```python
from build123d import *

# Parameters (mm, degrees)
SKETCH_1_W          = 20
SKETCH_1_H          = 20
EXTRUDE_1_DEPTH     = 50
SKETCH_2_R          = 1.5
CUT_EXTRUDE_1_DEPTH = 20
SKETCH_4_R          = 1.5
CUT_EXTRUDE_3_DEPTH = 20


with BuildPart() as part:
    # 草图1 → 凸台-拉伸1 (new body)
    with BuildSketch(Plane.XY):
        Rectangle(SKETCH_1_W, SKETCH_1_H)
    extrude(amount=EXTRUDE_1_DEPTH)

    # 草图2 → 切除-拉伸1 (cut)
    with BuildSketch(Plane(origin=(10, 0, 0), x_dir=(0, 0, -1), z_dir=(1, 0, 0))):
        with Locations((-32.5, 5.05)):
            Circle(SKETCH_2_R)
        with Locations((-17.5, 5.05)):
            Circle(SKETCH_2_R)
        with Locations((-32.5, -4.95)):
            Circle(SKETCH_2_R)
        with Locations((-17.5, -4.95)):
            Circle(SKETCH_2_R)
    extrude(amount=-CUT_EXTRUDE_1_DEPTH, mode=Mode.SUBTRACT)

    # 草图4 → 切除-拉伸3 (cut)
    with BuildSketch(Plane.XZ.offset(10)):
        with Locations(Location((-4.85, 40.893026958, 0), (0, 0, 270))):
            Circle(SKETCH_4_R)
        with Locations(Location((-4.85, 24.893026958, 0), (0, 0, 270))):
            Circle(SKETCH_4_R)
        with Locations(Location((-4.85, 8.893026958, 0), (0, 0, 270))):
            Circle(SKETCH_4_R)
        with Locations(Location((4.85, 8.893026958, 0), (0, 0, 270))):
            Circle(SKETCH_4_R)
        with Locations(Location((4.85, 24.893026958, 0), (0, 0, 270))):
            Circle(SKETCH_4_R)
        with Locations(Location((4.85, 40.893026958, 0), (0, 0, 270))):
            Circle(SKETCH_4_R)
    extrude(amount=-CUT_EXTRUDE_3_DEPTH, mode=Mode.SUBTRACT)


solid = part.part
```
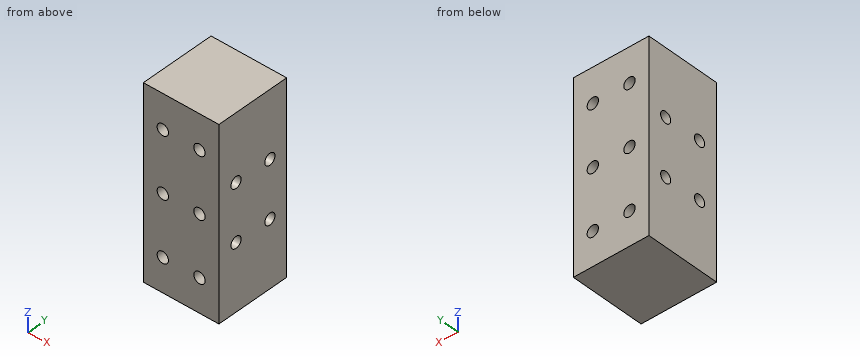
The listing builds one solid part. Answer for the finished solid, in the listing's coordinates (mm). Coordinates: 2 decimals unless noted, no trailing zeros. Write each loop counter-clockwise with the first axis right and the second up, starting at its lowest first coordinate (ties: lowest second). Pieces come first, ordered by that corner, then holes. Notation, with made-up numbers: (18.5, 66) -> (40.5, 66) arc R9 cw to (40.5, 70) -> close; hole circle Ø6 at (-30.5, 73). An arc over 180 degrees is marked (long way). Write each question's results on one line, items separated by ' | '. Start each with the question number.
1) Straight lines are drawn through the part: probe 1 along Y at (x, z) = (4.25, 17.5); probe 2 along X at (y, z) = (-8.75, 9); probe 3 along X at (y, z) = (-5.5, 10). For each, find the intervals that lie inside material, in ascending order.
2) Flat-ended cylindrical pins translate along their axes: pin 1 Ø2.5 at (x, z) = (4.85, 24.89) entering from -Y; pin 2 Ø3.5 at (x, z) = (4.85, 40.89) entering from +Y. Find the tip coordinate at first contact, or state that the pin passes through.
3) A cutting plane is placed at C-C (z = 17.5). Determine the outline of the cut face in (x, y).
4) A cutting plane is placed at B-B (x = -4.25). Determine the outline of the cut face in (y, z).
5) A cutting plane is placed at D-D (y = -1). Determine the outline of the cut face in (x, z), then the cut area to 3 significant figures.
6) A cutting plane is placed at A-A (y = 5.05). Count the separate pieces of the cut face and the enclosed holes in it, then the cut area to 3 significant figures.
Values follow:
1) probe 1: -10 to -6.45, -3.45 to 3.55, 6.55 to 10 | probe 2: -10 to -6.35, -3.35 to 3.35, 6.35 to 10 | probe 3: -10 to -5.86, -3.84 to 3.84, 5.86 to 10
2) pin 1: through | pin 2: y = 10
3) outline: (-10, -10) -> (10, -10) -> (10, -6.45) -> (-10, -6.45) -> close; (-10, -3.45) -> (10, -3.45) -> (10, 3.55) -> (-10, 3.55) -> close; (-10, 6.55) -> (10, 6.55) -> (10, 10) -> (-10, 10) -> close
4) outline: (-10, 0) -> (10, 0) -> (10, 7.52) -> (-10, 7.52) -> close; (-10, 10.27) -> (10, 10.27) -> (10, 23.52) -> (-10, 23.52) -> close; (-10, 26.27) -> (10, 26.27) -> (10, 39.52) -> (-10, 39.52) -> close; (-10, 42.27) -> (10, 42.27) -> (10, 50) -> (-10, 50) -> close; hole circle Ø3 at (-4.95, 17.5); hole circle Ø3 at (-4.95, 32.5); hole circle Ø3 at (5.05, 17.5); hole circle Ø3 at (5.05, 32.5)
5) outline: (-10, 0) -> (10, 0) -> (10, 50) -> (-10, 50) -> close; hole circle Ø3 at (-4.85, 8.89); hole circle Ø3 at (-4.85, 24.89); hole circle Ø3 at (-4.85, 40.89); hole circle Ø3 at (4.85, 8.89); hole circle Ø3 at (4.85, 24.89); hole circle Ø3 at (4.85, 40.89) | area: 958 mm²
6) separate pieces: 3 | enclosed holes: 6 | area: 838 mm²
